Design review of the part shown in the three views and the two pictorial views. Dimensions are in mm from the part's minimum x, y and z. A direction names the side the tool comes from. Give positions to 0.01 mm unless a question says otherwise; leave off trailing zeros. Write each loop counter-clockwise with the first axis right and the second up, starting at its lowest first coordinate (ties: lowest second). Pieces come first, ordered by that corner, then holes. Notation, with made-up numbers: M 26,-15.5 L 42,-15.5 A30 ccw 42,9.5 Z; hole C 61.5,85 d7. An arc over 180 degrees is marked long. Write item = value, one per line.
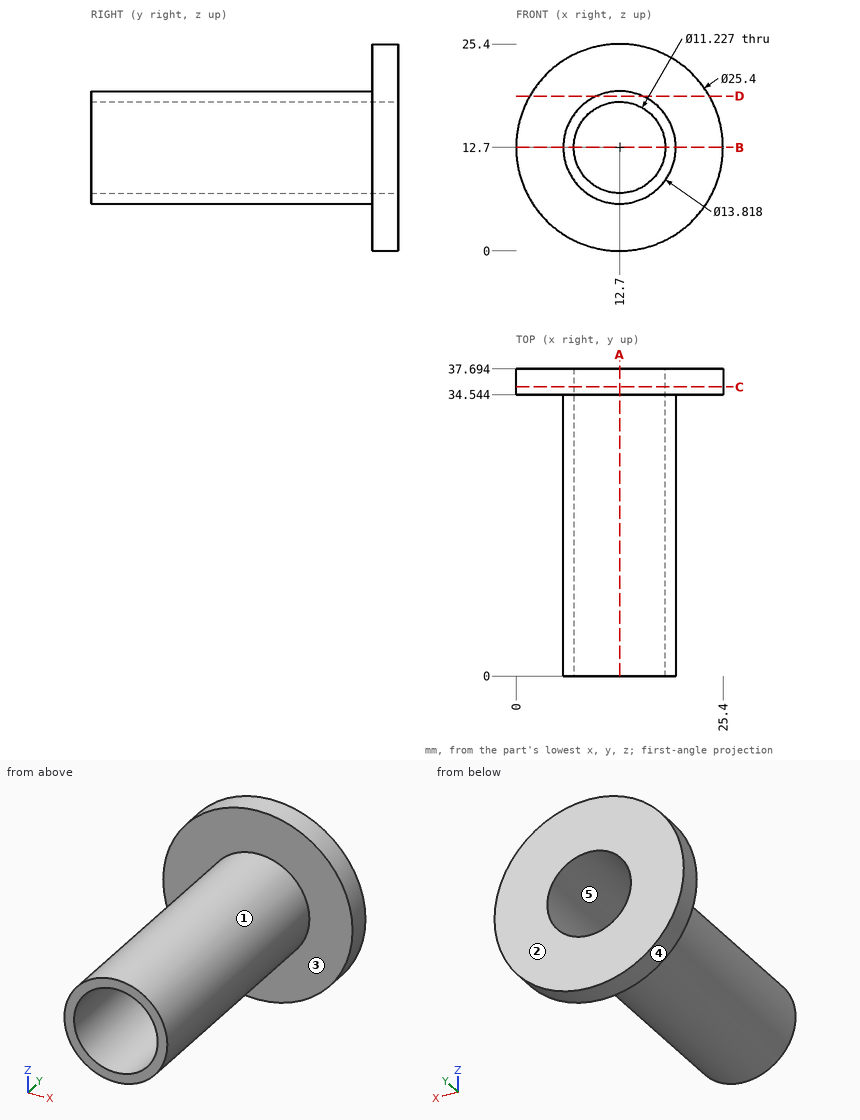
1. We need section B-B, the plane z = 12.7. Write out the cut boundary in (x, y).
Responses:
outline = M 0,34.54 L 5.79,34.54 L 5.79,0 L 7.09,0 L 7.09,37.69 L 0,37.69 Z; M 18.31,0 L 19.61,0 L 19.61,34.54 L 25.4,34.54 L 25.4,37.69 L 18.31,37.69 Z
2. We need section A-A, the plane x = 12.7. Write out the cut boundary in (y, z).
Responses:
outline = M 0,5.79 L 34.54,5.79 L 34.54,0 L 37.69,0 L 37.69,7.09 L 0,7.09 Z; M 0,18.31 L 37.69,18.31 L 37.69,25.4 L 34.54,25.4 L 34.54,19.61 L 0,19.61 Z
3. We need section C-C, the plane y = 35.5. Write out the cut boundary in (x, z).
Responses:
outline = C 12.7,12.7 d25.4; hole C 12.7,12.7 d11.23
4. Insertion check: P1, Ø3, axis at x = 14, y = 31.5, coming from the +Z side; P2, Ø2, axis at y = 15.5, z = 19, coming from the -X side; P3, Ø10, axis at y = 20.5, z = 22.5, coming from the +X side; P4, Ø9, axis at x = 12.7, z = 12.7, coming from the +Y side. Each pin has a flat end and moves straight along its axis. Give the tip position at first contact, or say it passes through.
Responses:
P1 = 19.61
P2 = 8.27
P3 = 17.67
P4 = through
5. We need section D-D, the plane z = 19. Write out the cut boundary in (x, y) (1 decimal), then the cut area to 3 significant figures.
Responses:
outline = M 1.7,34.5 L 9.9,34.5 L 9.9,0 L 15.5,0 L 15.5,34.5 L 23.7,34.5 L 23.7,37.7 L 1.7,37.7 Z
area = 265 mm2
6. For line 1 along Z through (x, y) = (12.7, 14.5); line 2 along Z through (x, y) = (9, 6.5) (1 decimal); line 3 along Y through (x, z) = (2.25, 13.25), list the stretches that pass through material, from the lowest coordinate up. Write a range as from..to.
Responses:
line_1 = 5.79..7.09, 18.31..19.61
line_2 = 6.9..8.5, 16.9..18.5
line_3 = 34.54..37.69
7. Machinability: for the marked faces 1 and 2, which of the approach directions +Z, -Z, +X, -X, +Y, -Y give a long, thin tool a straight path to every point of the face, cutting with its end or side? Answer none if there is none.
Responses:
face_1 = -Y
face_2 = +Z, -Z, +X, -X, +Y
8. The part is to be moulded in two halves that separate along Z. For the marked faces 3, 4 and 5, say which applies: +Z half, -Z half, draft (parallel to the pull), parting line (faces both ways), or undercut.
Responses:
face_3 = draft
face_4 = parting line
face_5 = undercut
